The listing builds one solid part. Answer for the finished solid, in the listing's coordinates (mm). A direction names the side the tool comes from. Coordinates: 2 decimals unless noted, no trailing zeros. Order: outer loops, then holes, each group sorted by start corner. A loop starts at its lowest first (then second) coordinate and runs counter-clockwise, first axis right, second up. Notation, with made-up numbers: (88.5, -1) -> (117.5, -1) arc R11 cw to (117.5, 13) -> close; hole circle Ø2 at (-13.75, 14). An arc over 180 degrees is marked (long way). Return JSON: item names as keys, results as strings.
```python
from build123d import *


with BuildPart() as part:
    # Sketch1 → Revolve1 (revolve)
    with BuildSketch(Plane.XY):
        with BuildLine():
            Line((-5.1562, 3.2385), (4.144991846, 3.2385))
            Line((4.144991846, 3.2385), (5.1562, 4.0005))
            Line((5.1562, 4.0005), (5.1562, 4.4831))
            ThreePointArc((5.1562, 4.4831), (5.044607684, 4.752507684), (4.7752, 4.8641))
            Line((4.7752, 4.8641), (1.9558, 4.8641))
            ThreePointArc((1.9558, 4.8641), (1.686392316, 4.752507684), (1.5748, 4.4831))
            Line((1.5748, 4.4831), (1.5748, 3.7719))
            Line((1.5748, 3.7719), (-5.1562, 3.7719))
            Line((-5.1562, 3.7719), (-5.1562, 3.2385))
        make_face()
    revolve(axis=Axis((-5.1562, 0, 0), (1, 0, 0)))


solid = part.part
```
Item 1: Which of the six approach directions +Z, -Z, +X, -X, +Y, -Y give full straight-line access (tool end or side, diameter ignored) to faces 1 (the cylindrical face through (3.35, -1.05, -4.75)), 2 (the flat face through (1.575, -4, -1))?
Answer list:
{"face 1": "+X, -X", "face 2": "-X"}
Item 2: The part is cut by section C-C on x = -0.75. Determine the outline of the cut face in (y, z), plus the area to 3 significant figures.
Answer list:
{"outline": "circle Ø7.54 at (0, 0); hole circle Ø6.48 at (0, 0)", "area": "11.7 mm2"}
Item 3: Flat-ended cylindrical pins translate along their axes: pin 1 (3 mm diameter, centred on x = -0.5, y = 0, fed in from -Z); pin 2 (3 mm diameter, centred on y = 4, z = 3.5, fed in from -X); pin 3 (1.5 mm diameter, centred on x = -2.5, y = -1, fed in from +Z). Find the tip coordinate at first contact, or state that the pin passes through.
Answer list:
{"pin 1": "z = -3.77", "pin 2": "x = 1.57", "pin 3": "z = 3.76"}
Item 4: The part is cut by section D-D on x = 3.5. Determine the outline of the cut face in (y, z).
Answer list:
{"outline": "circle Ø9.73 at (0, 0); hole circle Ø6.48 at (0, 0)"}
Item 5: Determine the mould class of faces 3 (the flat face through (-5.156, 2, 3)), 4 (the cylindrical face through (-0.44, -0.7, -3.16)), 5 (the cylindrical face through (-1.84, -2.99, -2.3)) for opening direction Y: pulls with the +Y half, pulls with the -Y half, needs draft (parallel to the pull), parting line crosses it, or undercut.
Answer list:
{"face 3": "needs draft", "face 4": "undercut", "face 5": "parting line crosses it"}
Item 6: The part is cut by section A-A on z = 0. Determine the outline of the cut face in (x, y) (1 decimal), plus the area to 3 significant figures.
Answer list:
{"outline": "(-5.2, -3.8) -> (1.6, -3.8) -> (1.6, -4.5) arc R0.4 ccw to (2, -4.9) -> (4.8, -4.9) arc R0.4 ccw to (5.2, -4.5) -> (5.2, -4) -> (4.1, -3.2) -> (-5.2, -3.2) -> close; (-5.2, 3.2) -> (4.1, 3.2) -> (5.2, 4) -> (5.2, 4.5) arc R0.4 ccw to (4.8, 4.9) -> (2, 4.9) arc R0.4 ccw to (1.6, 4.5) -> (1.6, 3.8) -> (-5.2, 3.8) -> close", "area": "17.9 mm2"}
Item 7: Find the intervals of material crossed by probe 1 along Z at (x, y) = (-0.5, 0); probe 2 along Z at (x, y) = (2, 0); probe 3 along Y at (x, z) = (-0.25, -2.75), in increasing order.
Answer list:
{"probe 1": "-3.77 to -3.24, 3.24 to 3.77", "probe 2": "-4.86 to -3.24, 3.24 to 4.86", "probe 3": "-2.58 to -1.71, 1.71 to 2.58"}
